from build123d import *

# Parameters (mm, degrees)
F0_R         = 4
F1_DEPTH     = 8.5
F2_R         = 8
F4_DEPTH     = 29
F5_R         = 4
F6_DEPTH     = 35
F7_W         = 22
F7_H         = 75.6632985204
F8_DEPTH     = 72.001
F9_DEPTH     = 35
F10_T1_DEPTH = 80.2241965153
F10_T3_DEPTH = 17.8781354595
F10_T5_DEPTH = 16.8781354595
F10_T7_DEPTH = 25.8982236505
F10_T9_DEPTH = 24.8982236505


# Not quite as in the source:
# - a fillet or chamfer that OpenCascade refuses, or shapes differently, is made with other operations: its cross-section is extruded or revolved along the edge and cut away or added


with BuildPart() as f1:
    # F0 (on Top) → F1 (new body)
    with BuildSketch(Plane.XY):
        with BuildLine():
            Line((0, 68), (0, 0))
            Line((0, 0), (35, 0))
            Line((35, 0), (35, 68))
            Line((35, 68), (35, 81))
            ThreePointArc((35, 81), (32.3639610307, 87.3639610307), (26, 90))
            Line((26, 90), (12, 90))
            Line((12, 90), (0, 68))
        make_face()
        with Locations((26, 81)):
            Circle(F0_R, mode=Mode.SUBTRACT)
        Polygon((35, 0), (0, 0), (-12, -31), (-12, -37), (6, -57), (35, -57), align=None)
        with Locations((-3, -33.8997244835)):
            Circle(F0_R, mode=Mode.SUBTRACT)
    extrude(amount=F1_DEPTH)

    # F2
    f2_edges = [f1.edges().sort_by_distance(p)[0] for p in [
        (-12, -37, 4.25),
        (-12, -31, 4.25),
    ]]
    fillet(f2_edges, radius=F2_R)

    # F3 (on face) → F4 (join, through all)
    with BuildSketch(Plane.YZ.offset(35)):
        Polygon((-57, 10), (-57, 0), (-34, 0), (-34, 14.5), align=None)
    extrude(amount=-F4_DEPTH)

    # F5 (on face) → F6 (join, through all)
    with BuildSketch(Plane.YZ.offset(35)):
        with BuildLine():
            Line((-23, 20), (-23, 8.5))
            Line((-23, 8.5), (67.7691474557, 8.5))
            ThreePointArc((67.7691474557, 8.5), (66.7805333738, 41.7873112781), (52.7728251344, 72))
            Line((52.7728251344, 72), (3.4575131106, 50))
            Line((3.4575131106, 50), (-23, 20))
        make_face()
        with Locations((13, 23)):
            Circle(F5_R, mode=Mode.SUBTRACT)
    extrude(amount=-F6_DEPTH)

    # F7 (on Top) → F8 (cut, through all)
    with BuildSketch(Plane.XY):
        with Locations((17, 14.7745097056)):
            Rectangle(F7_W, F7_H)
    extrude(amount=F8_DEPTH, mode=Mode.SUBTRACT)

    # F5 (on face) → F9 (join, through all)
    with BuildSketch(Plane.YZ.offset(35)):
        with Locations((13, 23)):
            Circle(F5_R)
    extrude(amount=-F9_DEPTH)

    # F10: fillet of radius 10 on 5 edges, made by hand

    # F10_s2 → F10_t1 (cut)
    with BuildSketch(Plane.YZ.offset(-22.6120982577)):
        with BuildLine():
            ThreePointArc((57.7430836083, 64.4431720463), (52.1704386948, 68.9292292294), (45.0268385832, 68.5444463974))
            Line((45.0268385832, 68.5444463974), (52.7728251344, 72))
            ThreePointArc((52.7728251344, 72), (55.3610878115, 68.2894186982), (57.7430836083, 64.4431720463))
        make_face()
    extrude(amount=F10_T1_DEPTH, mode=Mode.SUBTRACT)

    # F10_s4 → F10_t3 (cut)
    with BuildSketch(Plane.YZ.offset(22.5609322702)):
        with BuildLine():
            ThreePointArc((5.4443969789, 50.886366593), (3.5960570103, 49.8115072456), (2.0184710529, 48.3682796811))
            Line((2.0184710529, 48.3682796811), (3.4575131106, 50))
            Line((3.4575131106, 50), (5.4443969789, 50.886366593))
        make_face()
    extrude(amount=F10_T3_DEPTH, mode=Mode.SUBTRACT)

    # F10_s6 → F10_t5 (cut)
    with BuildSketch(Plane.YZ.offset(-5.4390677298)):
        with BuildLine():
            ThreePointArc((5.4443969789, 50.886366593), (3.5960570103, 49.8115072456), (2.0184710529, 48.3682796811))
            Line((2.0184710529, 48.3682796811), (3.4575131106, 50))
            Line((3.4575131106, 50), (5.4443969789, 50.886366593))
        make_face()
    extrude(amount=F10_T5_DEPTH, mode=Mode.SUBTRACT)

    # F10_s8 → F10_t7 (cut)
    with BuildSketch(Plane.YZ.offset(18.5508881748)):
        with BuildLine():
            ThreePointArc((-23, 16.2203552699), (-22.3541434669, 19.7558891758), (-20.5, 22.8347335476))
            Line((-20.5, 22.8347335476), (-23, 20))
            Line((-23, 20), (-23, 16.2203552699))
        make_face()
    extrude(amount=F10_T7_DEPTH, mode=Mode.SUBTRACT)

    # F10_s10 → F10_t9 (cut)
    with BuildSketch(Plane.YZ.offset(-9.4491118252)):
        with BuildLine():
            ThreePointArc((-20.5, 22.8347335476), (-22.3541434669, 19.7558891758), (-23, 16.2203552699))
            Line((-23, 16.2203552699), (-23, 20))
            Line((-23, 20), (-20.5, 22.8347335476))
        make_face()
    extrude(amount=F10_T9_DEPTH, mode=Mode.SUBTRACT)


solid = f1.part
Geometry check sheet. Reference: the model listing, model coordinates, mm. A direction names the side the tool comes from. Round coordinates to 2 decimals unless told otherwise and drop trailing zeros. Write each loop counter-clockwise with the first axis right and the second up, starting at its lowest first coordinate (ties: lowest second). Pieces come first, ordered by that corner, then holes. Notation, with made-up numbers: (87, 84) -> (103, 84) arc R24 cw to (103, 119) -> close; hole circle Ø4 at (5, 16). An arc over 180 degrees is marked (long way). One line per item, written item: value. Start each with the question number.
(1) Cross-section at B-B, the plane x = -3. Record the cut outline in (y, z).
(2) Access from +Z, -Z, +X, -X, +Y, -Y to the whole of each face (thin tool, end or side, straight path). Record for faces 4 (the flat face through (3, -23, 12)), 5 (the flat face through (19, 90, 4)), 6 (the flat face through (21, -34, 11)), 7 (the flat face through (1, 18, 0)), 8 (the flat face through (17, -23.057, 4)).
(3) Cross-section at A-A, the plane x = 13.5. Record the cut outline in (y, z).
(4) Scan lines: line 1 (Y direction, x = 26, z = 2); line 2 (X direction, y = 42.5, z = 20.5); line 3 (X direction, y = 58.5, z = 31). Record each from-to range of solid material in increasing order. Write a range as [from, to].
(5) Go/stop test with flat-tipped pins: pin 1 Ø12 at (x, z) = (-4, 41) entering from +Y; pin 2 Ø6.5 at (x, y) = (22, 81.5) entering from +Z; pin 3 Ø8 at (x, y) = (28.5, -15) entering from +Z. Record where each tip stops, or that it passes through.
(6) Cross-section at C-C, the plane z = 13. Record the cut outline in (x, y), and give its area (3 significant figures).
(7) Draft check along Z on faces 1 (the cylindrical face through (2.958, -22.336, 19.803)), 2 (the cylindrical face through (-3.521, -29.934, 4.19)), 3 (the cylindrical face through (17.74, 67.77, 36.96)). Enter one of: +Z half, -Z half, draft (parallel to the pull), parting line (faces both ways), or undercut.
(8) Cross-section at D-D, the plane z = 54.5. Record the cut outline in (x, y).
Answer:
1. outline: (-47, 0) -> (-37.9, 0) -> (-37.9, 8.5) -> (-47, 8.5) -> close; (-29.9, 0) -> (-7.75, 0) -> (-7.75, 8.5) -> (-29.9, 8.5) -> close
2. face 4: +Z, +X, -X, -Y
2. face 5: +Z, -Z, +X, -X, +Y
2. face 6: +Z, +X, -X
2. face 7: -Z, +X, -X, +Y, -Y
2. face 8: +Z, -Z
3. outline: (-57, 0) -> (-23.06, 0) -> (-23.06, 8.5) -> (-34, 8.5) -> (-34, 14.5) -> (-57, 10) -> close; circle Ø8 at (13, 23); (52.61, 0) -> (90, 0) -> (90, 8.5) -> (67.77, 8.5) arc R82.9 ccw to (57.74, 64.44) arc R10 ccw to (52.61, 68.78) -> close
4. line 1: [-57, -23.06], [52.61, 77], [85, 90]
4. line 2: [0, 6], [28, 35]
4. line 3: [0, 35]
5. pin 1: y = 67.84
5. pin 2: z = 8.5
5. pin 3: z = 33.61
6. outline: (0, -23) -> (6, -23) -> (6, 52.61) -> (28, 52.61) -> (28, -23) -> (35, -23) -> (35, 68.43) -> (0, 68.43) -> close; (6, -41.67) -> (35, -41.67) -> (35, -34) -> (6, -34) -> close
6. area: 1,760 mm²
7. face 1: +Z half
7. face 2: draft
7. face 3: undercut
8. outline: (0, 13.54) -> (6, 13.54) -> (6, 52.61) -> (28, 52.61) -> (28, 13.54) -> (35, 13.54) -> (35, 62.67) -> (0, 62.67) -> close
